Geometry check sheet. Reference: the model listing, model coordinates, mm. A direction names the side the tool comes from. Round coordinates to 2 decimals unless told otherwise and drop trailing zeros. Loops run counter-clockwise (first coordinate to the right, second up) from the corner with the lowest first, then second, coordinate; pieces in that order, holes last. Notation, with made-up numbers: (-4.75, 61.5) -> (19.25, 61.5) arc R24 ccw to (19.25, 98.5) -> close; hole circle Ø5 at (-40, 7). An arc over 180 degrees is marked (long way). Use one line per item in the form item = value.
from build123d import *

# Parameters (mm, degrees)
F0_W     = 31.8
F0_H     = 31.8
F1_DEPTH = 9.6
F2_W     = 29.4
F2_H     = 29.4
F3_DEPTH = 8.4
F4_R     = 2


# Not quite as in the source:
# - a feature names something its author has since deleted; it is built from what else it names


with BuildPart() as f1:
    # F0 (on Top) → F1 (new body)
    with BuildSketch(Plane.XY):
        Rectangle(F0_W, F0_H)
    extrude(amount=F1_DEPTH)

    # F2 (on Top) → F3 (cut)
    with BuildSketch(Plane.XY):
        Rectangle(F2_W, F2_H)
    extrude(amount=F3_DEPTH, mode=Mode.SUBTRACT)

    # F4
    f4_edges = [f1.edges().sort_by_distance(p)[0] for p in [
        (-15.9, -15.9, 4.8),
        (-15.9, 15.9, 4.8),
        (15.9, 15.9, 4.8),
        (15.9, -15.9, 4.8),
    ]]
    fillet(f4_edges, radius=F4_R)


solid = f1.part
1. Section check B-B (x = -8). Record the boundary of the cut face in (y, z).
Return value:
outline = (-15.9, 0) -> (-14.7, 0) -> (-14.7, 8.4) -> (14.7, 8.4) -> (14.7, 0) -> (15.9, 0) -> (15.9, 9.6) -> (-15.9, 9.6) -> close
2. Section check A-A (z = 6.25). Record the boundary of the cut face in (x, y).
Return value:
outline = (-15.9, -13.9) arc R2 ccw to (-13.9, -15.9) -> (13.9, -15.9) arc R2 ccw to (15.9, -13.9) -> (15.9, 13.9) arc R2 ccw to (13.9, 15.9) -> (-13.9, 15.9) arc R2 ccw to (-15.9, 13.9) -> close; hole (-14.7, -14.7) -> (14.7, -14.7) -> (14.7, 14.7) -> (-14.7, 14.7) -> close
3. Tool access check on faces 4 (the flat face through (0, 14.7, 4)), 5 (the cylindrical face through (-15.33, -15.3, 4.87)). Record the directions out of +Z, -Z, +X, -X, +Y, -Y that give a thin tool (end or side, any length) a straight path to the whole face; none if there is none.
Return value:
face_4 = -Z
face_5 = +Z, -Z, -X, -Y
4. Gauge pin test, flat end, axial feed: pin 1 (10 mm diameter, centred on x = -4, y = -1.5, fed in from -Z). Record the tip position at first contact, or that the pin passes through.
Return value:
pin_1 = 8.4
5. Mould release check, pull along Y, two halves, no side actions. Record for faces 1 (the cylindrical face through (-15.33, 15.3, 4.87)), 2 (the flat face through (-14.7, 0, 4)), 3 (the flat face through (0, -15, 0)): released by +Y, released by -Y, zero draft, split by the parting line, or undercut.
Return value:
face_1 = released by +Y
face_2 = undercut
face_3 = zero draft
6. Material ranges on line 1 along Y through (x, z) = (-8.5, 4.5); line 2 along X through (y, z) = (14, 8.5), recorded low to high.
Return value:
line_1 = -15.9 to -14.7, 14.7 to 15.9
line_2 = -15.9 to 15.9
